from build123d import *

# Parameters (mm, degrees)
SKETCH1_W           = 118.618
SKETCH1_H           = 50.8
BOSS_EXTRUDE1_DEPTH = 31.75
SKETCH2_R           = 5.715
BOSS_EXTRUDE2_DEPTH = 17.78
CUT_EXTRUDE1_DEPTH  = 9.906


with BuildPart() as part:
    # Sketch1 → Boss-Extrude1 (new body)
    with BuildSketch(Plane(origin=(0, 0, 0), x_dir=(1, 0, 0), z_dir=(0, 1, 0))):
        Rectangle(SKETCH1_W, SKETCH1_H)
    extrude(amount=BOSS_EXTRUDE1_DEPTH)

    # Sketch2 → Boss-Extrude2 (add)
    with BuildSketch(Plane(origin=(59.309, 0, 0), x_dir=(0, 0, -1), z_dir=(1, 0, 0))):
        with Locations((0, 15.875)):
            Circle(SKETCH2_R)
    extrude(amount=BOSS_EXTRUDE2_DEPTH)

    # Sketch3 → Cut-Extrude1 (cut)
    with BuildSketch(Plane.ZY.offset(59.309)):
        with BuildLine():
            Line((-7.963952601, 11.6586), (-2.54, 11.6586))
            Line((-2.54, 11.6586), (0, 14.1986))
            Line((0, 14.1986), (2.54, 11.6586))
            Line((2.54, 11.6586), (7.963952601, 11.6586))
            ThreePointArc((7.963952601, 11.6586), (10.210514576, 15.875), (7.963952601, 20.0914))
            Line((7.963952601, 20.0914), (2.54, 20.0914))
            Line((2.54, 20.0914), (0, 17.5514))
            Line((0, 17.5514), (-2.54, 20.0914))
            Line((-2.54, 20.0914), (-7.963952601, 20.0914))
            ThreePointArc((-7.963952601, 20.0914), (-10.210514576, 15.875), (-7.963952601, 11.6586))
        make_face()
    extrude(amount=-CUT_EXTRUDE1_DEPTH, mode=Mode.SUBTRACT)


solid = part.part
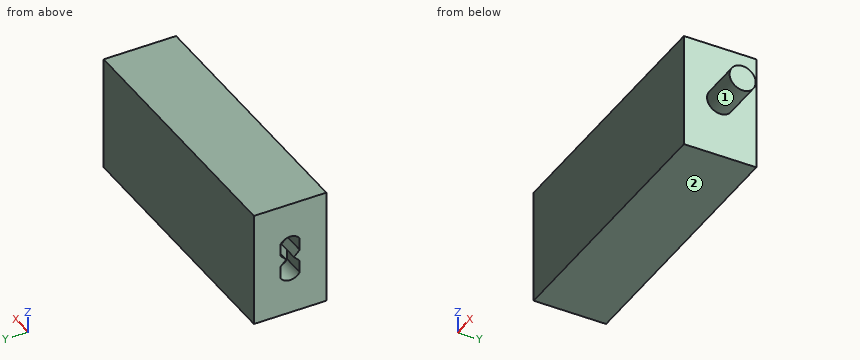
For this review, take the finished solid that the model builds, in its own axes (mm). Face numbers are marked on the shaded views. A direction names the side the tool comes from. Round coordinates to 2 decimals unless told otherwise and drop trailing zeros. Order: outer loops, then holes, each group sorted by start corner. A loop starts at its lowest first (then second) coordinate and runs counter-clockwise, first axis right, second up. Notation, with made-up numbers: M -28.5,23 L 6.5,23 A16 ccw 6.5,51 Z; hole C 37.5,40 d10. An arc over 180 degrees is marked long. Use a Markdown table: item, result. Add a question column.
Item 1: To check wall thickness, follow line 1 along X through (y, z) = (15, -22.5); line 2 along Z through (x, y) = (67, 16); line 3 along Y through (x, z) = (64, -4). State the ranges of each line that lie inside material, in increasing order.
Item 2: Add section B-B, the plane z = -17.5. Give the boundary of the cut face in (x, y).
Item 3: Tool access review of the marked faces 1 and 2: name each direction out of +Z, -Z, +X, -X, +Y, -Y from which nothing blocks a thin tool from reaching the whole face with its end or side.
Item 4: Add section A-A, the plane y = 4. Give the boundary of the cut face in (x, z), then the cut area to 3 significant figures.
Geometry results:
| question | item | result |
|---|---|---|
| 1 | line 1 | x = -59.31 to 59.31 |
| 1 | line 2 | z = -5.71 to 5.71 |
| 1 | line 3 | y = 11.79 to 19.96 |
| 2 | outline | M -59.31,0 L 59.31,0 L 59.31,31.75 L -59.31,31.75 Z |
| 3 | face 1 | +X |
| 3 | face 2 | -Z, +X, -X, +Y, -Y |
| 4 | outline | M -59.31,-25.4 L 59.31,-25.4 L 59.31,25.4 L -59.31,25.4 Z |
| 4 | area | 6,030 mm² |
